```python
from build123d import *

# Parameters (mm, degrees)
SKETCH1_W           = 120.2
SKETCH1_H           = 120.2
SKETCH1_W_2         = 110.2
SKETCH1_H_2         = 110.2
BOSS_EXTRUDE1_DEPTH = 4
SKETCH2_W           = 10.1
SKETCH2_H           = 10.1
BOSS_EXTRUDE2_DEPTH = 2.3
SKETCH3_W           = 25
SKETCH3_H           = 25
SKETCH3_R           = 3
SKETCH3_W_2         = 24.35
SKETCH3_H_2         = 24.35
BOSS_EXTRUDE3_DEPTH = 4
FILLET1_R           = 12
SKETCH5_R           = 5.417288046
BOSS_EXTRUDE4_DEPTH = 10
CUT_EXTRUDE1_START  = -12.5
SKETCH4_W           = 6.076696642
SKETCH4_H           = 5
CUT_EXTRUDE1_DEPTH  = 10
CIRPATTERN1_COUNT   = 4
SKETCH6_R           = 22.094645404
CUT_EXTRUDE2_DEPTH  = 10
BOSS_EXTRUDE5_DEPTH = 2.3
SKETCH9_W           = 17.742485537
SKETCH9_H           = 24.263991122
SKETCH9_W_2         = 24.263991122
SKETCH9_H_2         = 17.742485537
CUT_EXTRUDE3_DEPTH  = 10


with BuildPart() as part:
    # Sketch1 → Boss-Extrude1 (new body)
    with BuildSketch(Plane(origin=(0, 0, 0), x_dir=(1, 0, 0), z_dir=(0, 1, 0))):
        Rectangle(SKETCH1_W, SKETCH1_H)
        Rectangle(SKETCH1_W_2, SKETCH1_H_2, mode=Mode.SUBTRACT)
    extrude(amount=BOSS_EXTRUDE1_DEPTH)

    # Sketch2 → Boss-Extrude2 (add)
    with BuildSketch(Plane(origin=(0, 4, 0), x_dir=(1, 0, 0), z_dir=(0, 1, 0))):
        with Locations((-50.05, 50.05)):
            Rectangle(SKETCH2_W, SKETCH2_H)
        with Locations((50.05, 50.05)):
            Rectangle(SKETCH2_W, SKETCH2_H)
        with Locations((50.05, -50.05)):
            Rectangle(SKETCH2_W, SKETCH2_H)
        with Locations((-50.05, -50.05)):
            Rectangle(SKETCH2_W, SKETCH2_H)
    extrude(amount=-BOSS_EXTRUDE2_DEPTH)

    # Sketch3 → Boss-Extrude3 (add)
    # profile 1 of 4: a face of its own
    with BuildSketch(Plane(origin=(0, 0, 0), x_dir=(-1, 0, 0), z_dir=(0, -1, 0))):
        with Locations((72.6, -47.6)):
            Rectangle(SKETCH3_W, SKETCH3_H)
        with Locations(Location((75.1, -50.1, 0), (0, 0, 90))):
            Circle(SKETCH3_R, mode=Mode.SUBTRACT)
    # profile 2 of 4: a face of its own
    with BuildSketch(Plane(origin=(0, 0, 0), x_dir=(-1, 0, 0), z_dir=(0, -1, 0))):
        with Locations((-72.6, -47.6)):
            Rectangle(SKETCH3_W, SKETCH3_H)
        with Locations(Location((-74.9, -50.1, 0), (0, 0, 90))):
            Circle(SKETCH3_R, mode=Mode.SUBTRACT)
    # profile 3 of 4: a face of its own
    with BuildSketch(Plane(origin=(0, 0, 0), x_dir=(-1, 0, 0), z_dir=(0, -1, 0))):
        with Locations((72.6, 47.6)):
            Rectangle(SKETCH3_W, SKETCH3_H)
        with Locations(Location((75.1, 49.9, 0), (0, 0, 90))):
            Circle(SKETCH3_R, mode=Mode.SUBTRACT)
    # profile 4 of 4: a face of its own
    with BuildSketch(Plane(origin=(0, 0, 0), x_dir=(-1, 0, 0), z_dir=(0, -1, 0))):
        with Locations((-72.275, 47.925)):
            Rectangle(SKETCH3_W_2, SKETCH3_H_2)
        with Locations(Location((-75.260238187, 49.598128293, 0), (0, 0, 90))):
            Circle(SKETCH3_R, mode=Mode.SUBTRACT)
    extrude(amount=-BOSS_EXTRUDE3_DEPTH)

    # Fillet1
    fillet1_edges = [part.edges().sort_by_distance(p)[0] for p in [
        (85.1, 2, 60.1),
        (85.1, 2, 35.1),
        (60.1, 2, 35.1),
        (84.45, 2, -60.1),
        (60.1, 2, -35.75),
        (84.45, 2, -35.75),
        (-60.1, 2, 35.1),
        (-85.1, 2, 35.1),
        (-85.1, 2, 60.1),
        (-60.1, 2, -35.1),
        (-85.1, 2, -60.1),
        (-85.1, 2, -35.1),
    ]]
    fillet(fillet1_edges, radius=FILLET1_R)

    # Sketch4 → Cut-Extrude1 (cut)
    with BuildSketch(Plane(origin=(0, 0, 0), x_dir=(-1, 0, 0), z_dir=(0, -1, 0)).offset(CUT_EXTRUDE1_START)):
        with BuildLine():
            Line((60.786291501, -27.1), (64.782340933, -27.1))
            Line((64.782340933, -27.1), (64.782340933, -21.023303358))
            Line((64.782340933, -21.023303358), (60.1, -21.023303358))
            Line((60.1, -21.023303358), (60.1, -23.1))
            ThreePointArc((60.1, -23.1), (60.272817284, -25.129223745), (60.786291501, -27.1))
        make_face()
        with BuildLine():
            Line((55.1, -27.1), (60.786291501, -27.1))
            ThreePointArc((60.786291501, -27.1), (60.272817284, -25.129223745), (60.1, -23.1))
            Line((60.1, -23.1), (60.1, -21.023303358))
            Line((60.1, -21.023303358), (55.1, -21.023303358))
            Line((55.1, -21.023303358), (55.1, -27.1))
        make_face()
        with Locations((24.061651679, -57.6)):
            Rectangle(SKETCH4_W, SKETCH4_H)
    cut_extrude1 = extrude(amount=CUT_EXTRUDE1_DEPTH, mode=Mode.SUBTRACT)

    # CirPattern1: Cut-Extrude1 ×4 about axis
    cirpattern1_axis = Axis((0, 0, 0), (0, 1, 0))
    for i in range(1, CIRPATTERN1_COUNT):
        add(cut_extrude1.rotate(cirpattern1_axis, i * 360 / CIRPATTERN1_COUNT), mode=Mode.SUBTRACT)

    # Sketch8 → Boss-Extrude5 (add)
    with BuildSketch(Plane(origin=(0, 1.7, 0), x_dir=(-1, 0, 0), z_dir=(0, -1, 0))):
        Polygon((50.704922644, -45), (9.738912133, -4.033989488), (4.033989488, -4.033989488), (4.033989488, -9.738912133), (45, -50.704922645), (45, -45), align=None)
        Polygon((4.033989488, -9.738912133), (0, -5.704922645), (-4.033989488, -9.738912133), (-4.033989488, -75.048460322), (4.033989488, -75.048460322), align=None)
        Polygon((-50.214813889, -55.919736534), (-4.033989488, -9.738912133), (-4.033989488, -4.033989488), (-9.738912133, -4.033989488), (-55.919736534, -50.214813889), align=None)
        Polygon((-9.738912133, -4.033989488), (-5.704922645, 0), (-9.738912133, 4.033989488), (-75.048460322, 4.033989488), (-75.048460322, -4.033989488), align=None)
        Polygon((-4.033989488, 4.033989488), (-4.033989488, 9.738912133), (-50.214813889, 55.919736534), (-55.919736534, 50.214813889), (-9.738912133, 4.033989488), align=None)
        Polygon((0, 5.704922645), (4.033989488, 9.738912133), (4.033989488, 75.048460322), (-4.033989488, 75.048460322), (-4.033989488, 9.738912133), align=None)
        Polygon((9.738912133, 4.033989488), (55.919736534, 50.214813889), (50.214813889, 55.919736534), (4.033989488, 9.738912133), (4.033989488, 4.033989488), align=None)
        Polygon((75.048460322, 4.033989488), (9.738912133, 4.033989488), (5.704922645, 0), (9.738912133, -4.033989488), (75.048460322, -4.033989488), align=None)
        Polygon((-4.033989488, -9.738912133), (0, -5.704922645), (-1.670933156, -4.033989488), (-4.033989488, -4.033989488), align=None)
        Polygon((4.033989488, -4.033989488), (1.670933156, -4.033989488), (0, -5.704922645), (4.033989488, -9.738912133), align=None)
        Polygon((9.738912133, -4.033989488), (5.704922645, 0), (4.033989488, -1.670933156), (4.033989488, -4.033989488), align=None)
        Polygon((5.704922645, 0), (9.738912133, 4.033989488), (4.033989488, 4.033989488), (4.033989488, 1.670933156), align=None)
        Polygon((1.670933156, 4.033989488), (4.033989488, 4.033989488), (4.033989488, 9.738912133), (0, 5.704922645), align=None)
        Polygon((-1.670933156, 4.033989488), (0, 5.704922645), (-4.033989488, 9.738912133), (-4.033989488, 4.033989488), align=None)
        Polygon((-5.704922645, 0), (-4.033989488, 1.670933156), (-4.033989488, 4.033989488), (-9.738912133, 4.033989488), align=None)
        Polygon((-9.738912133, -4.033989488), (-4.033989488, -4.033989488), (-4.033989488, -1.670933157), (-5.704922645, 0), align=None)
        Polygon((0, -5.704922645), (1.670933156, -4.033989488), (-1.670933156, -4.033989488), align=None)
        Polygon((4.033989488, -4.033989488), (4.033989488, -1.670933156), (1.670933156, -4.033989488), align=None)
        Polygon((4.033989488, -1.670933156), (5.704922645, 0), (4.033989488, 1.670933156), align=None)
        Polygon((4.033989488, 1.670933156), (4.033989488, 4.033989488), (1.670933156, 4.033989488), align=None)
        Polygon((-4.033989488, 1.670933156), (-1.670933156, 4.033989488), (-4.033989488, 4.033989488), align=None)
        Polygon((-4.033989488, -1.670933157), (-4.033989488, 1.670933156), (-5.704922645, 0), align=None)
        Polygon((-4.033989488, -4.033989488), (-1.670933156, -4.033989488), (-4.033989488, -1.670933157), align=None)
        Polygon((1.670933156, -4.033989488), (4.033989488, -1.670933156), (4.033989488, 1.670933156), (1.670933156, 4.033989488), (-1.670933156, 4.033989488), (-4.033989488, 1.670933156), (-4.033989488, -1.670933157), (-1.670933156, -4.033989488), align=None)
        Polygon((-1.670933156, 4.033989488), (1.670933156, 4.033989488), (0, 5.704922645), align=None)
    extrude(amount=-BOSS_EXTRUDE5_DEPTH)

    # Sketch9 → Cut-Extrude3 (cut)
    with BuildSketch(Plane(origin=(0, 1.7, 0), x_dir=(-1, 0, 0), z_dir=(0, -1, 0))):
        with Locations((1.428324636, -72.231995561)):
            Rectangle(SKETCH9_W, SKETCH9_H)
        with Locations((-72.231995561, -1.428324636)):
            Rectangle(SKETCH9_W_2, SKETCH9_H_2)
        with Locations((-1.428324636, 72.231995561)):
            Rectangle(SKETCH9_W, SKETCH9_H)
        with Locations((72.231995561, 1.428324636)):
            Rectangle(SKETCH9_W_2, SKETCH9_H_2)
    extrude(amount=-CUT_EXTRUDE3_DEPTH, mode=Mode.SUBTRACT)


with BuildPart() as body_2:
    # Sketch5 → Boss-Extrude4 (new body)
    with BuildSketch(Plane.XZ):
        with Locations(Location((0, 0, 0), (0, 0, 270))):
            Circle(SKETCH5_R)
    extrude(amount=BOSS_EXTRUDE4_DEPTH)

    # Sketch6 → Cut-Extrude2 (cut)
    with BuildSketch(Plane.XZ.offset(10)):
        Circle(SKETCH6_R)
    extrude(amount=-CUT_EXTRUDE2_DEPTH, mode=Mode.SUBTRACT)


solid = part.part
```
Verification items for the finished model (mm, model axes). A direction names the side the tool comes from. Round coordinates to 2 decimals unless told otherwise and drop trailing zeros. Write each loop counter-clockwise with the first axis right and the second up, starting at its lowest first coordinate (ties: lowest second). Pieces come first, ordered by that corner, then holes.
1. Section check A-A on x = 32.5. Enter the section's corners in (y, z).
2. Scan lines: L1, parallel to Z at x = 52, y = 1.2; L2, parallel to X at y = 2.2, z = -44.5; L3, parallel to Z at x = 51, y = 3.25. Record each from-to range of solid material in increasing order.
3. Access from +Z, -Z, +X, -X, +Y, -Y to the whole of each face (thin tool, end or side, straight path). Record for faces 1 (the flat face through (29.935, 2.834, 24.23)), 2 (the cylindrical face through (63.71, 2.03, 31.68)), 3 (the flat face through (58, 2.5, 24)).
4. Gauge pin test, flat ends, axial feed: P1, Ø2, axis at y = 3, z = -15.5, coming from the +X side; P2, Ø1.2, axis at y = 3.5, z = -58.5, coming from the +X side; P3, Ø0.7, axis at y = 3, z = -54, coming from the +X side; P4, Ø6.5, axis at x = -57.5, z = 23.5, coming from the +Y side. Record the tip position at first contact, or that the pin passes through.
5. Section check D-D on x = 67. Enter the section's corners in (y, z), plus the area to 3 significant figures.
6. Draft check along X on faces 4 (the flat face through (24.23, 2.834, -29.935)), 5 (the flat face through (-0.8, 1.5, 55.1)), 6 (the cylindrical face through (-81.49, 2.03, -56.68)), 7 (the flat face through (1, 4, -1)). Enter one of: +X half, -X half, draft (parallel to the pull), parting line (faces both ways), or undercut.
7. Section check B-B on z = -39. Enter the section's corners in (x, y).
8. Section check C-C on y = 0.8. State how many separate pieces and enclosed holes the cut face has, plus the area to 3 significant figures.
Answer:
1. outline: (0, -60.1) - (4, -60.1) - (4, -55.1) - (0, -55.1) - close; (0, 55.1) - (4, 55.1) - (4, 60.1) - (0, 60.1) - close; (1.7, -38.2) - (4, -38.2) - (4, -26.8) - (1.7, -26.8) - close; (1.7, -4.03) - (4, -4.03) - (4, 4.03) - (1.7, 4.03) - close; (1.7, 26.8) - (4, 26.8) - (4, 38.2) - (1.7, 38.2) - close
2. L1: z = -60.1 to -55.1, 55.1 to 60.1
2. L2: x = -84.81 to -55.1, -50.2 to -38.8, -4.03 to 4.03, 38.8 to 50.2, 55.1 to 84
2. L3: z = -60.1 to -45, -4.03 to 4.03, 45 to 60.1
3. face 1: +Y, -Y
3. face 2: +X, +Y, -Y
3. face 3: +Y
4. P1: stops at x = 60.1
4. P2: stops at x = 79.38
4. P3: stops at x = 83.09
4. P4: stops at y = 4
5. outline: (0, -60.1) - (4, -60.1) - (4, -34.61) - (0, -34.61) - close; (0, 33.96) - (4, 33.96) - (4, 60.1) - (0, 60.1) - close
5. area: 207 mm2
6. face 4: undercut
6. face 5: undercut
6. face 6: -X half
6. face 7: draft
7. outline: (-81.95, 0) - (-55.1, 0) - (-55.1, 4) - (-81.95, 4) - close; (-44.7, 1.7) - (-33.3, 1.7) - (-33.3, 4) - (-44.7, 4) - close; (-4.03, 1.7) - (4.03, 1.7) - (4.03, 4) - (-4.03, 4) - close; (33.3, 1.7) - (44.7, 1.7) - (44.7, 4) - (33.3, 4) - close; (55.1, 0) - (80.66, 0) - (80.66, 4) - (55.1, 4) - close
8. separate pieces: 1
8. enclosed holes: 5
8. area: 4,540 mm2
